Build history of the part. All positions in model axes, mm. A direction names the side the tool comes from. Give positions to 0.01 mm unless a question says otherwise; leave off trailing zeros. Write each loop counter-clockwise with the first axis right and the second up, starting at its lowest first coordinate (ties: lowest second). Pieces come first, ordered by that corner, then holes. Notation, with made-up numbers: M 29,13 L 86,13 A7 ccw 86,20 Z; hole C 28,43.25 d11. An arc over 180 degrees is marked long. Return JSON: item names as keys, results as strings. Group by question number.
Q1. Pull direction Y, two halves, no side cores. Call faces 4 (the flat face through (-5, -154, 3)), 5 (the flat face through (0, 2, 5)), 6 (the flat face through (11, -164, 2)): +Y half, -Y half, draft (parallel to the pull), parting line (faces both ways), or undercut.
Q2. Wall check: probe 1 along Y at (x, z) = (0, 1.2); probe 2 along Y at (x, z) = (-3.5, 1.1); probe 3 along Y at (x, z) = (1, 3.85). Give the ranges that are in metal, low to high.
Q3. Tool access for faces 1 (the flat face through (0, -149, 3)), 2 (the flat face through (-2.1, -162, 3)), 3 (the flat face through (-2.1, 161, 3)): list every direction of +Z, -Z, +X, -X, +Y, -Y with a clear straight run to the whole face (end or side of a thin tool).
Q4. Band-saw the part on A-A, the plane z = 0.75. Give the cut face in (x, y) (3 decimals), then the cut area to 3 significant figures.
from build123d import *

# Parameters (mm, degrees)
SKETCH1_W           = 40.89
SKETCH1_H           = 328
BOSS_EXTRUDE1_DEPTH = 5
SKETCH2_R           = 2.1
CUT_EXTRUDE1_DEPTH  = 10
CUT_EXTRUDE2_DEPTH  = 10
SKETCH4_R           = 2.1
CUT_EXTRUDE3_DEPTH  = 5
SKETCH5_R           = 2.1
CUT_EXTRUDE4_DEPTH  = 5


with BuildPart() as part:
    # Sketch1 → Boss-Extrude1 (new body)
    with BuildSketch(Plane.XY):
        Rectangle(SKETCH1_W, SKETCH1_H)
    extrude(amount=BOSS_EXTRUDE1_DEPTH)

    # Sketch2 → Cut-Extrude1 (cut)
    with BuildSketch(Plane.XY.offset(5)):
        with Locations((0, -81.5)):
            Circle(SKETCH2_R)
    extrude(amount=-CUT_EXTRUDE1_DEPTH, mode=Mode.SUBTRACT)

    # Sketch3 → Cut-Extrude2 (cut)
    with BuildSketch(Plane.XY.offset(5)):
        Polygon((-2.1, -164), (-2.1, -159), (-5, -159), (-5, -149), (5, -149), (5, -159), (2.1, -159), (2.1, -164), align=None)
        Polygon((2.1, 164), (2.1, 159), (5, 159), (5, 149), (-5, 149), (-5, 159), (-2.1, 159), (-2.1, 164), align=None)
    extrude(amount=-CUT_EXTRUDE2_DEPTH, mode=Mode.SUBTRACT)

    # Sketch4 → Cut-Extrude3 (cut)
    with BuildSketch(Plane.XY.offset(5)):
        with Locations((0, -106.5)):
            Circle(SKETCH4_R)
    extrude(amount=-CUT_EXTRUDE3_DEPTH, mode=Mode.SUBTRACT)

    # Sketch5 → Cut-Extrude4 (cut)
    with BuildSketch(Plane.XY.offset(5)):
        with Locations((0, 11.5)):
            Circle(SKETCH5_R)
    extrude(amount=-CUT_EXTRUDE4_DEPTH, mode=Mode.SUBTRACT)


solid = part.part
From the geometry:
{
 "1": {"face 4": "undercut", "face 5": "draft", "face 6": "-Y half"},
 "2": {"probe 1": "y = -149 to -108.6, -104.4 to -83.6, -79.4 to 9.4, 13.6 to 149", "probe 2": "y = -164 to -159, -149 to 149, 159 to 164", "probe 3": "y = -149 to -108.35, -104.65 to -83.35, -79.65 to 9.65, 13.35 to 149"},
 "3": {"face 1": "+Z, -Z", "face 2": "+Z, -Z, -Y", "face 3": "+Z, -Z, +Y"},
 "4": {"outline": "M -20.445,-164 L -2.1,-164 L -2.1,-159 L -5,-159 L -5,-149 L 5,-149 L 5,-159 L 2.1,-159 L 2.1,-164 L 20.445,-164 L 20.445,164 L 2.1,164 L 2.1,159 L 5,159 L 5,149 L -5,149 L -5,159 L -2.1,159 L -2.1,164 L -20.445,164 Z; hole C 0,-106.5 d4.2; hole C 0,-81.5 d4.2; hole C 0,11.5 d4.2", "area": "13,100 mm^2"}
}
